```python
from build123d import *

# Parameters (mm, degrees)
SKETCH_1_W          = 38
SKETCH_1_H          = 55
EXTRUDE_1_DEPTH     = 3
SKETCH_2_W          = 3
SKETCH_2_H          = 36
SKETCH_2_H_2        = 1.5
CUT_EXTRUDE_1_DEPTH = 3
SKETCH_3_R          = 1.5
CUT_EXTRUDE_2_DEPTH = 4
SKETCH_4_W          = 4
SKETCH_4_H          = 9
CUT_EXTRUDE_3_DEPTH = 10
SKETCH_5_W          = 1.5
SKETCH_5_H          = 12
EXTRUDE_2_DEPTH     = 3
SKETCH_6_R          = 0.5
CUT_EXTRUDE_4_DEPTH = 10


with BuildPart() as part:
    # 草图1 → 凸台-拉伸1 (new body)
    with BuildSketch(Plane.XY):
        Rectangle(SKETCH_1_W, SKETCH_1_H)
    extrude(amount=EXTRUDE_1_DEPTH)

    # 草图2 → 切除-拉伸1 (cut)
    with BuildSketch(Plane.XY.offset(3)):
        with Locations((-17.5, 0)):
            Rectangle(SKETCH_2_W, SKETCH_2_H)
        with Locations((-17.5, 26.75)):
            Rectangle(SKETCH_2_W, SKETCH_2_H_2)
        with Locations((17.5, -26.75)):
            Rectangle(SKETCH_2_W, SKETCH_2_H_2)
        with Locations((17.5, 0)):
            Rectangle(SKETCH_2_W, SKETCH_2_H)
        with Locations((17.5, 26.75)):
            Rectangle(SKETCH_2_W, SKETCH_2_H_2)
        with Locations((-17.5, -26.75)):
            Rectangle(SKETCH_2_W, SKETCH_2_H_2)
    extrude(amount=-CUT_EXTRUDE_1_DEPTH, mode=Mode.SUBTRACT)

    # 草图3 → 切除-拉伸2 (cut, through all)
    with BuildSketch(Plane.XY.offset(3)):
        with Locations((-13.75, -22)):
            Circle(SKETCH_3_R)
        with Locations((13.75, -22)):
            Circle(SKETCH_3_R)
        with Locations((13.75, 22)):
            Circle(SKETCH_3_R)
        with Locations((-13.75, 22)):
            Circle(SKETCH_3_R)
    extrude(amount=-CUT_EXTRUDE_2_DEPTH, mode=Mode.SUBTRACT)

    # 草图4 → 切除-拉伸3 (cut)
    with BuildSketch(Plane.XY.offset(3)):
        with Locations((8, -16)):
            Rectangle(SKETCH_4_W, SKETCH_4_H)
        with Locations((0, -16)):
            Rectangle(SKETCH_4_W, SKETCH_4_H)
        with Locations((-8, -16)):
            Rectangle(SKETCH_4_W, SKETCH_4_H)
        with Locations((-8, 16)):
            Rectangle(SKETCH_4_W, SKETCH_4_H)
        with Locations((8, 16)):
            Rectangle(SKETCH_4_W, SKETCH_4_H)
        with Locations((0, 16)):
            Rectangle(SKETCH_4_W, SKETCH_4_H)
    extrude(amount=-CUT_EXTRUDE_3_DEPTH, mode=Mode.SUBTRACT)

    # 草图5 → 凸台-拉伸2 (add, through all)
    with BuildSketch(Plane.XY.offset(3)):
        with Locations((-16.75, 0)):
            Rectangle(SKETCH_5_W, SKETCH_5_H)
        with Locations((16.75, 0)):
            Rectangle(SKETCH_5_W, SKETCH_5_H)
    extrude(amount=-EXTRUDE_2_DEPTH)

    # 草图6 → 切除-拉伸4 (cut)
    with BuildSketch(Plane.XY.offset(3)):
        with Locations((-16.212132034, -26.212132034)):
            Circle(SKETCH_6_R)
        with Locations((-16.212132034, -17.787867966)):
            Circle(SKETCH_6_R)
        with Locations((-16.212132034, -6.212132034)):
            Circle(SKETCH_6_R)
        with Locations((16.212132034, -6.212132034)):
            Circle(SKETCH_6_R)
        with Locations((16.212132034, -17.787867966)):
            Circle(SKETCH_6_R)
        with Locations((16.212132034, -26.212132034)):
            Circle(SKETCH_6_R)
        with Locations((16.212132034, 26.212132034)):
            Circle(SKETCH_6_R)
        with Locations((16.212132034, 17.787867966)):
            Circle(SKETCH_6_R)
        with Locations((16.212132034, 6.212132034)):
            Circle(SKETCH_6_R)
        with Locations((-16.212132034, 6.212132034)):
            Circle(SKETCH_6_R)
        with Locations((-16.212132034, 17.787867966)):
            Circle(SKETCH_6_R)
        with Locations((-16.212132034, 26.212132034)):
            Circle(SKETCH_6_R)
    extrude(amount=-CUT_EXTRUDE_4_DEPTH, mode=Mode.SUBTRACT)


solid = part.part
```
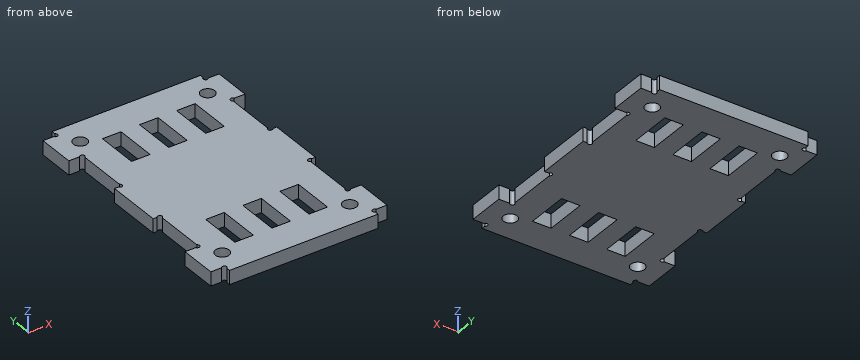
Here's how the part is built. I have some questions about the finished solid (model axes, mm). Give positions to 0.01 mm unless a question says otherwise; leave off trailing zeros. Write each loop counter-clockwise with the first axis right and the second up, starting at its lowest first coordinate (ties: lowest second). Pieces come first, ordered by that corner, then holes. Notation, with made-up numbers: M 5.5,28 L 61.5,28 A16 ccw 61.5,55 Z; hole C 68,16 d4. An arc over 180 degrees is marked long. Put each result on its own line as item: value. Start each with the question number.
Item 1: I need wall thicknesses on L1, parallel to Y at x = 1, z = 2.1; L2, parallel to Y at x = 13.75, z = 0.9; L3, parallel to X at y = 9, z = 1.75. Which ranges of each line are inside material? Lowest first, please. Write a range as from..to.
Item 2: If we section it at D-D, the plane z = 0.45: Count the separate pieces of the cut face and the enclosed holes in it, then the cut area to 3 significant figures.
Item 3: If we section it at B-B, the plane y = 15.5: Write out the boundary of the cut face in (x, z), then the cut area to 3 significant figures.
Item 4: If we section it at C-C, the plane x = -13.75: Write out the boundary of the cut face in (y, z), then the cut area to 3 significant figures.
Item 5: Will these pins go through, and if not, where does the flat tip stop? pin 1 (1.8 mm diameter, centred on x = 13.75, y = 22, fed in from -Z); pin 2 (1.5 mm diameter, centred on y = 1.5, z = 1.5, fed in from +X); pin 3 (1.5 mm diameter, centred on y = 14.5, z = 1, fed in from -X); pin 4 (0.7 mm diameter, centred on x = 17.5, z = 1, fed in from +Y).
Item 6: If we section it at A-A, the plane y = 22: Write out the boundary of the cut face in (x, z), then the cut area to 3 significant figures.
Values:
1. L1: -27.5..-20.5, -11.5..11.5, 20.5..27.5
1. L2: -27.5..-23.5, -20.5..20.5, 23.5..27.5
1. L3: -16..16
2. separate pieces: 1
2. enclosed holes: 10
2. area: 1,640 mm²
3. outline: M -16,0 L -10,0 L -10,3 L -16,3 Z; M -6,0 L -2,0 L -2,3 L -6,3 Z; M 2,0 L 6,0 L 6,3 L 2,3 Z; M 10,0 L 16,0 L 16,3 L 10,3 Z
3. area: 60.0 mm²
4. outline: M -27.5,0 L -23.5,0 L -23.5,3 L -27.5,3 Z; M -20.5,0 L 20.5,0 L 20.5,3 L -20.5,3 Z; M 23.5,0 L 27.5,0 L 27.5,3 L 23.5,3 Z
4. area: 147 mm²
5. pin 1: through
5. pin 2: x = 17.5
5. pin 3: x = -16
5. pin 4: y = 26
6. outline: M -19,0 L -15.25,0 L -15.25,3 L -19,3 Z; M -12.25,0 L 12.25,0 L 12.25,3 L -12.25,3 Z; M 15.25,0 L 19,0 L 19,3 L 15.25,3 Z
6. area: 96.0 mm²
